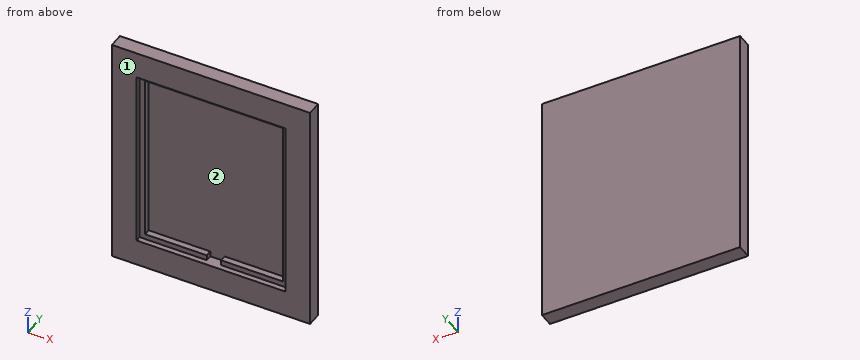
from build123d import *

# Parameters (mm, degrees)
F0_W     = 110
F0_H     = 130
F1_DEPTH = 8
F2_W     = 82.5
F2_H     = 100.5
F3_DEPTH = 3
F4_W     = 8
F4_H     = 3
F5_DEPTH = 3.5


with BuildPart() as f1:
    # F0 (on Front) → F1 (new body)
    with BuildSketch(Plane.XZ):
        with Locations((-4.093055, 2.210701)):
            Rectangle(F0_W, F0_H)
    extrude(amount=F1_DEPTH)

    # F2 (on face) → F3 (cut)
    with BuildSketch(Plane.XZ.offset(8)):
        with Locations((-4.093055, 2.210701)):
            Rectangle(F2_W, F2_H)
    extrude(amount=-F3_DEPTH, mode=Mode.SUBTRACT)

    # F4 (on face) → F5 (cut)
    with BuildSketch(Plane.XZ.offset(5)):
        Polygon((34.156945, 49.460701), (-42.343055, 49.460701), (-42.343055, -45.039299), (-8.093055, -45.039299), (-0.093055, -45.039299), (34.156945, -45.039299), align=None)
        with Locations((-4.093055, -46.539299)):
            Rectangle(F4_W, F4_H)
    extrude(amount=-F5_DEPTH, mode=Mode.SUBTRACT)


solid = f1.part
CAD build for the part. Positions are in the model's coordinates, mm. Face numbers are marked on the shaded views. Give positions to 0.01 mm unless a question says otherwise; leave off trailing zeros. Write each loop counter-clockwise with the first axis right and the second up, starting at its lowest first coordinate (ties: lowest second). Pieces come first, ordered by that corner, then holes. Notation, with made-up numbers: (50, -37.75) -> (96, -37.75) arc R23 ccw to (96, 1.25) -> close; hole circle Ø6 at (-11, -14). An arc over 180 degrees is marked (long way). Return JSON: item names as keys, results as strings.
Item 1: Band-saw the part on A-A (y = -3.75). List the corners of the cut face in (x, z).
Answer below:
{"outline": "(-59.09, -62.79) -> (50.91, -62.79) -> (50.91, 67.21) -> (-59.09, 67.21) -> close; hole (-42.34, -45.04) -> (-8.09, -45.04) -> (-8.09, -48.04) -> (-0.09, -48.04) -> (-0.09, -45.04) -> (34.16, -45.04) -> (34.16, 49.46) -> (-42.34, 49.46) -> close"}
Item 2: Band-saw the part on C-C (x = 29.5). List the corners of the cut face in (y, z).
Answer below:
{"outline": "(-8, -62.79) -> (0, -62.79) -> (0, 67.21) -> (-8, 67.21) -> (-8, 52.46) -> (-5, 52.46) -> (-5, 49.46) -> (-1.5, 49.46) -> (-1.5, -45.04) -> (-5, -45.04) -> (-5, -48.04) -> (-8, -48.04) -> close"}
Item 3: Band-saw the part on B-B (z = 25.5). List the corners of the cut face in (x, y).
Answer below:
{"outline": "(-59.09, -8) -> (-45.34, -8) -> (-45.34, -5) -> (-42.34, -5) -> (-42.34, -1.5) -> (34.16, -1.5) -> (34.16, -5) -> (37.16, -5) -> (37.16, -8) -> (50.91, -8) -> (50.91, 0) -> (-59.09, 0) -> close"}
Item 4: Two-plate mould, pull along X, no slides. Class the marked faces 1 and 2: +X half, -X half, draft (parallel to the pull), parting line (faces both ways), or undercut.
Answer below:
{"face 1": "draft", "face 2": "undercut"}
Item 5: Drill centre lines: probe 1 along X at (y, z) = (-6, -34.5); probe 2 along Z at (x, y) = (-36.5, -6); probe 3 along X at (y, z) = (-2.5, -47.5). Where is each one in solid material? Low to high.
Answer below:
{"probe 1": "x = -59.09 to -45.34, 37.16 to 50.91", "probe 2": "z = -62.79 to -48.04, 52.46 to 67.21", "probe 3": "x = -59.09 to -8.09, -0.09 to 50.91"}
Item 6: Drop a flat-ended pin along its axis: pin 1 (25 mm diameter, centred on x = -8.5, z = -19.5, fed in from -Y). Give the stop position or say it passes through.
Answer below:
{"pin 1": "stops at y = -1.5"}
